```python
from build123d import *

# Parameters (mm, degrees)
BOSS_EXTRU_1_DEPTH      = 5
BOSS_EXTRU_2_DEPTH      = 15
BOSS_EXTRU_3_DEPTH      = 15
ESQUISSE5_W             = 2.4467389
ESQUISSE5_H             = 15
ESQUISSE5_W_2           = 2.875
ESQUISSE5_W_3           = 2.123659042
ESQUISSE5_H_2           = 5
ESQUISSE5_W_4           = 1.985062281
BOSS_EXTRU_4_DEPTH      = 2.5
ESQUISSE6_W             = 33.5
ESQUISSE6_H             = 3
ENL_V_MAT_EXTRU_1_DEPTH = 2.5
ESQUISSE8_W             = 5
ESQUISSE8_H             = 2
BOSS_EXTRU_5_DEPTH      = 1
ESQUISSE9_W             = 5
ESQUISSE9_H             = 12
BOSS_EXTRU_6_DEPTH      = 1


with BuildPart() as part:
    # Esquisse1 → Boss.-Extru.1 (new body)
    with BuildSketch(Plane.XY):
        with BuildLine():
            Line((0.5, -4.5), (0, -4.5))
            Line((0, -4.5), (0, -5))
            Line((0, -5), (0.5, -5))
            Line((0.5, -5), (2, -5))
            Line((2, -5), (3.75, -2.9))
            Line((3.75, -2.9), (41.25, -2.9))
            Line((41.25, -2.9), (43, -5))
            Line((43, -5), (44.5, -5))
            Line((44.5, -5), (45, -5))
            Line((45, -5), (45, -4.5))
            Line((45, -4.5), (44.5, -4.5))
            ThreePointArc((44.5, -4.5), (42.5, -2.5), (44.5, -0.5))
            Line((44.5, -0.5), (45, -0.5))
            Line((45, -0.5), (45, 0))
            Line((45, 0), (44.5, 0))
            Line((44.5, 0), (39.25, 0))
            Line((39.25, 0), (39.25, -0.5))
            Line((39.25, -0.5), (40.625, -2.15))
            Line((40.625, -2.15), (4.375, -2.15))
            Line((4.375, -2.15), (5.75, -0.5))
            Line((5.75, -0.5), (5.75, 0))
            Line((5.75, 0), (0, 0))
            Line((0, 0), (0, -0.5))
            Line((0, -0.5), (0.5, -0.5))
            ThreePointArc((0.5, -0.5), (2.5, -2.5), (0.5, -4.5))
        make_face()
    extrude(amount=BOSS_EXTRU_1_DEPTH)

    # Esquisse3 → Boss.-Extru.2 (add)
    with BuildSketch(Plane.XY.offset(5)):
        Polygon((40.25, -2.9), (39.625, -2.15), (5.375, -2.15), (4.75, -2.9), align=None)
    extrude(amount=BOSS_EXTRU_2_DEPTH)

    # Esquisse4 → Boss.-Extru.3 (add)
    with BuildSketch(Plane.XY.offset(20)):
        with BuildLine():
            Line((0.5, -4.5), (0, -4.5))
            Line((0, -4.5), (0, -5))
            Line((0, -5), (0.5, -5))
            Line((0.5, -5), (2, -5))
            Line((2, -5), (3.75, -2.9))
            Line((3.75, -2.9), (41.25, -2.9))
            Line((41.25, -2.9), (43, -5))
            Line((43, -5), (44.5, -5))
            Line((44.5, -5), (45, -5))
            Line((45, -5), (45, -4.5))
            Line((45, -4.5), (44.5, -4.5))
            ThreePointArc((44.5, -4.5), (42.5, -2.5), (44.5, -0.5))
            Line((44.5, -0.5), (45, -0.5))
            Line((45, -0.5), (45, 0))
            Line((45, 0), (43.697090933, 0))
            Line((43.697090933, 0), (39.25, 0))
            Line((39.25, 0), (39.25, -0.5))
            Line((39.25, -0.5), (40.625, -2.15))
            Line((40.625, -2.15), (4.375, -2.15))
            Line((4.375, -2.15), (5.75, -0.5))
            Line((5.75, -0.5), (5.75, 0))
            Line((5.75, 0), (0, 0))
            Line((0, 0), (0, -0.5))
            Line((0, -0.5), (0.5, -0.5))
            ThreePointArc((0.5, -0.5), (2.5, -2.5), (0.5, -4.5))
        make_face()
    extrude(amount=BOSS_EXTRU_3_DEPTH)

    # Esquisse5 → Boss.-Extru.4 (add)
    with BuildSketch(Plane(origin=(0, 0, 0), x_dir=(1, 0, 0), z_dir=(0, 1, 0))):
        with Locations((40.47336945, -27.5)):
            Rectangle(ESQUISSE5_W, ESQUISSE5_H)
        with Locations((4.3125, -27.5)):
            Rectangle(ESQUISSE5_W_2, ESQUISSE5_H)
        with Locations((4.688170479, -2.5)):
            Rectangle(ESQUISSE5_W_3, ESQUISSE5_H_2)
        with Locations((40.242531141, -2.5)):
            Rectangle(ESQUISSE5_W_4, ESQUISSE5_H_2)
    extrude(amount=-BOSS_EXTRU_4_DEPTH)

    # Esquisse6 → Enlèv. mat.-Extru.1 (cut)
    with BuildSketch(Plane(origin=(0, -2.15, 0), x_dir=(1, 0, 0), z_dir=(0, 1, 0))):
        with Locations((22.5, -28.5)):
            Rectangle(ESQUISSE6_W, ESQUISSE6_H)
        with Locations((22.5, -23.5)):
            Rectangle(ESQUISSE6_W, ESQUISSE6_H)
    extrude(amount=-ENL_V_MAT_EXTRU_1_DEPTH, mode=Mode.SUBTRACT)

    # Esquisse8 → Boss.-Extru.5 (add)
    with BuildSketch(Plane(origin=(0, -2.15, 0), x_dir=(1, 0, 0), z_dir=(0, 1, 0))):
        with Locations((32.75, -26)):
            Rectangle(ESQUISSE8_W, ESQUISSE8_H)
        with Locations((12.25, -26)):
            Rectangle(ESQUISSE8_W, ESQUISSE8_H)
    extrude(amount=BOSS_EXTRU_5_DEPTH)

    # Esquisse9 → Boss.-Extru.6 (add)
    with BuildSketch(Plane(origin=(0, -1.15, 0), x_dir=(1, 0, 0), z_dir=(0, 1, 0))):
        with Locations((32.75, -21)):
            Rectangle(ESQUISSE9_W, ESQUISSE9_H)
        with Locations((12.25, -21)):
            Rectangle(ESQUISSE9_W, ESQUISSE9_H)
    extrude(amount=BOSS_EXTRU_6_DEPTH)


solid = part.part
```
Check sheet for the modelled part. Datum: model origin and axes. Units: mm. A direction names the side the tool comes from. Coordinates: 2 decimals unless noted, no trailing zeros. Loops run counter-clockwise (first coordinate to the right, second up) from the corner with the lowest first, then second, coordinate; pieces in that order, holes last.
1) Sectioned sample at A-A (x = 15.5). Record the boundary of the cut face in (y, z), and give its area (4 significant figures).
2) Sectioned sample at B-B (z = 15.5). Record the boundary of the cut face in (x, y) (3 decimals).
3) Sectioned sample at C-C (z = 4). Record the boundary of the cut face in (x, y), and give its area (3 significant figures).
4) Release check for a two-part mould opening along X. For faces 1 (the face through (12, -1.15, 20)), 2 (the face through (42.5, -2.5, 27.4)), 3 (the face through (1, -5, 2)), 4 (the face through (23, -2.15, 32)) record: released by +X, released by -X, zero draft, split by the parting line, or undercut.
5) Material ranges on probe 1 along Z at (x, y) = (27.5, -2.2); probe 2 along Y at (x, z) = (36.5, 33); probe 3 along Z at (x, y) = (41, -1.5), recorded low to high.
6) Gauge pin test, flat ends, axial feed: pin 1 (2 mm diameter, centred on x = 31.5, z = 29.5, fed in from +Y); pin 2 (5 mm diameter, centred on x = 11.5, z = 15.5, fed in from +Y); pin 3 (0.6 mm diameter, centred on y = -1.5, z = 3, fed in from +X). Record the tip position at first contact, or that the pin passes through.
7) Access from +Z, -Z, +X, -X, +Y, -Y to the whole of each face (thin tool, end or side, straight path). Record for faces 5 (the face through (42.113, -3.935, 27.395)), 6 (the face through (41, -2, 20)), 7 (the face through (22.3, -2.5, 27)).
8) Sectioned sample at D-D (x = 33). Record the boundary of the cut face in (y, z).
Check sheet entries:
1. outline: (-2.9, 0) - (-2.15, 0) - (-2.15, 22) - (-2.9, 22) - close; (-2.9, 25) - (-2.15, 25) - (-2.15, 27) - (-2.9, 27) - close; (-2.9, 30) - (-2.15, 30) - (-2.15, 35) - (-2.9, 35) - close
1. area: 21.75 mm2
2. outline: (4.75, -2.9) - (40.25, -2.9) - (39.625, -2.15) - (5.375, -2.15) - close; (9.75, -1.15) - (14.75, -1.15) - (14.75, -0.15) - (9.75, -0.15) - close; (30.25, -1.15) - (35.25, -1.15) - (35.25, -0.15) - (30.25, -0.15) - close
3. outline: (0, -5) - (2, -5) - (3.75, -2.9) - (41.25, -2.9) - (43, -5) - (45, -5) - (45, -4.5) - (44.5, -4.5) arc R2 cw to (44.5, -0.5) - (45, -0.5) - (45, 0) - (39.25, 0) - (39.25, -2.15) - (5.75, -2.15) - (5.75, 0) - (0, 0) - (0, -0.5) - (0.5, -0.5) arc R2 cw to (0.5, -4.5) - (0, -4.5) - close
3. area: 54.0 mm2
4. face 1: undercut
4. face 2: released by +X
4. face 3: zero draft
4. face 4: undercut
5. probe 1: z = 0 to 22, 25 to 27, 30 to 35
5. probe 2: y = -2.9 to -2.15
5. probe 3: z = 0 to 5, 20 to 35
6. pin 1: stops at y = -2.15
6. pin 2: stops at y = -0.15
6. pin 3: stops at x = 42.98
7. face 5: +Z, -Z, -Y
7. face 6: +X, +Y
7. face 7: +Y, -Y
8. outline: (-2.9, 0) - (-2.15, 0) - (-2.15, 22) - (-2.9, 22) - close; (-2.9, 25) - (-1.15, 25) - (-1.15, 15) - (-0.15, 15) - (-0.15, 27) - (-2.9, 27) - close; (-2.9, 30) - (-2.15, 30) - (-2.15, 35) - (-2.9, 35) - close
